Solid Edge part; units mm, degrees
sketch "Sketch1" plane through (0, 0, 0) normal (0, -1, 0) x (1, 0, 0)
  line L0 (0, 6) -> (1.5359, 6)
  line L1 (1.5359, 6) -> (5, 0)
  line L2 (5, 0) -> (0, 0)
  line L3 (0, 0) -> (0, 6)
revolve "RevolvedProtrusion1" add sketch "Sketch1" angle 360 about axis through (0, 0, 54) along (0, 0, -1)
sketch "Sketch2" plane through (0, 0, 0) normal (0, 0, -1) x (1, 0, 0)
  circle A0 centre (0, 0) radius 5
extrude "Protrusion1" add sketch "Sketch2" along normal blind 2
sketch "Sketch3" plane through (0, 0, -2) normal (0, 0, -1) x (1, 0, 0)
  circle A0 centre (0, 0) radius 3
extrude "ExtrudedProtrusion_2" add sketch "Sketch3" along normal blind 10
fillet "Round_1" radius 2 1 edges at (-3, 0, -2)
properties material "Stainless steel"
Can you work these out from the model? Positions are in its coordinate system, mm. A direction names the side the tool comes from. Coordinates: 2 decimals unless noted, no trailing zeros. Loops run counter-clockwise (first coordinate to the right, second up) from the corner with the lowest first, then second, coordinate; pieces in that order, holes last. Notation, with made-up numbers: M 63,68.25 L 120,68.25 A18 cw 120,102.25 Z; hole C 24,-17.5 d5. An arc over 180 degrees is marked long. Return JSON: item names as keys, results as strings. Group by question number.
Item 1: Imagine slicing it at C-C (z = -10.25). Please give me the cut outline in (x, y).
Item 2: If I drill on L1, parallel to X at y = 2, z = -6.5; L2, parallel to Y at x = 2.25, z = -1.5; L3, parallel to Z at x = -1.25, y = -3.25, over which ranges is the centre line in solid material (lowest first)? Write a range as from..to.
Item 3: Imagine slicing it at D-D (z = 5). Please give me the cut outline in (x, y).
Item 4: On a 3-axis mill with a long thin cutter (end or side, diameter ignored), from which of +Z, -Z, +X, -X, +Y, -Y can I reach the whole of each face in a straight line? I mean faces 1 (the cylindrical face through (-3, 0, -8)), 2 (the cylindrical face through (-1.08, -4.88, -0.99)). Say none if no direction works.
Item 5: I'm going to push flat-ended pins straight in: pin 1 Ø6 at (x, z) = (3, -0.5) entering from -Y; pin 2 Ø6 at (x, z) = (2.5, -6.5) entering from +Y; pin 3 Ø1 at (x, y) = (-4, 3) entering from -Z; pin 4 Ø5 at (x, z) = (-2, -4) entering from +Y. Where does each tip first touch, or does it pass through?
Verdict:
{
 "1": {"outline": "C 0,0 d6"},
 "2": {"L1": "x = -2.24..2.24", "L2": "y = -4.47..4.47", "L3": "z = -2.7..2.63"},
 "3": {"outline": "C 0,0 d4.23"},
 "4": {"face 1": "-Z", "face 2": "+Z, -Z"},
 "5": {"pin 1": "stops at y = -5", "pin 2": "stops at y = 3", "pin 3": "stops at z = -2.06", "pin 4": "stops at y = 4.97"}
}
